```python
from build123d import *

# Parameters (mm, degrees)
SKETCH2_W           = 70
SKETCH2_H           = 140
SKETCH2_R           = 1.5
BOSS_EXTRUDE1_DEPTH = 3.175
SKETCH3_R           = 1.75
CUT_EXTRUDE1_DEPTH  = 79.326755486


with BuildPart() as part:
    # Sketch2 → Boss-Extrude1 (new body)
    with BuildSketch(Plane(origin=(0, 0, 0), x_dir=(1, 0, 0), z_dir=(0, 1, 0))):
        Rectangle(SKETCH2_W, SKETCH2_H)
        with Locations(Location((31, -62, 0), (0, 0, 270))):
            Circle(SKETCH2_R, mode=Mode.SUBTRACT)
        with Locations(Location((31, 62, 0), (0, 0, 90))):
            Circle(SKETCH2_R, mode=Mode.SUBTRACT)
        with Locations(Location((-31, 62, 0), (0, 0, 270))):
            Circle(SKETCH2_R, mode=Mode.SUBTRACT)
        with Locations(Location((-31, -62, 0), (0, 0, 90))):
            Circle(SKETCH2_R, mode=Mode.SUBTRACT)
    extrude(amount=BOSS_EXTRUDE1_DEPTH)

    # Sketch3 → Cut-Extrude1 (cut, through all)
    with BuildSketch(Plane(origin=(0, 3.175, 0), x_dir=(1, 0, 0), z_dir=(0, 1, 0))):
        with Locations(Location((-24.999549753, -44.6, 0), (0, 0, 270))):
            Circle(SKETCH3_R)
        with Locations(Location((24, -44.810057195, 0), (0, 0, 270))):
            Circle(SKETCH3_R)
        with Locations(Location((24, 13.189942805, 0), (0, 0, 90))):
            Circle(SKETCH3_R)
        with Locations(Location((-24.999549753, 12.97988561, 0), (0, 0, 90))):
            Circle(SKETCH3_R)
    extrude(amount=-CUT_EXTRUDE1_DEPTH, mode=Mode.SUBTRACT)


solid = part.part
```
Check sheet for the modelled part. Datum: model origin and axes. Units: mm. Round coordinates to 2 decimals unless told otherwise and drop trailing zeros. Loops run counter-clockwise (first coordinate to the right, second up) from the corner with the lowest first, then second, coordinate; pieces in that order, holes last. Notation, with made-up numbers: (78, 17.25) -> (120, 17.25) arc R20 ccw to (120, 43.25) -> close; hole circle Ø7 at (49, 22.25). An arc over 180 degrees is marked (long way). Answer in a Markdown table with one row per item.
Q1. Release check for a two-part mould opening along X. For faces 1 (the face through (0, 3.175, -1)), 2 (the face through (-35, 2, 1)), 3 (the face through (-25.67, 1.61, 46.217)), 4 (the face through (-23.29, 1.61, -12.6)) record: released by +X, released by -X, zero draft, split by the parting line, or undercut.
Data:
| item | result |
|---|---|
| face 1 | zero draft |
| face 2 | released by -X |
| face 3 | undercut |
| face 4 | undercut |
Q2. Sectioned sample at B-B on z = 62. Enter the section's corners in (x, y) (3 decimals).
Data:
| item | result |
|---|---|
| outline | (-35, 0) -> (-32.5, 0) -> (-32.5, 3.175) -> (-35, 3.175) -> close; (-29.5, 0) -> (29.5, 0) -> (29.5, 3.175) -> (-29.5, 3.175) -> close; (32.5, 0) -> (35, 0) -> (35, 3.175) -> (32.5, 3.175) -> close |
Q3. Thickness scan on L1, parallel to X at y = 1.4, z = 44.6; L2, parallel to X at y = 1.8, z = -62; L3, parallel to Z at x = -25, y = 0.85. Record the ranges inside material, lowest first.
Data:
| item | result |
|---|---|
| L1 | x = -35 to -26.75, -23.25 to 22.26, 25.74 to 35 |
| L2 | x = -35 to -32.5, -29.5 to 29.5, 32.5 to 35 |
| L3 | z = -70 to -14.73, -11.23 to 42.85, 46.35 to 70 |
Q4. Sectioned sample at A-A on x = 31. Enter the section's corners in (y, z) (3 decimals), then the cut area to 3 significant figures.
Data:
| item | result |
|---|---|
| outline | (0, -70) -> (3.175, -70) -> (3.175, -63.5) -> (0, -63.5) -> close; (0, -60.5) -> (3.175, -60.5) -> (3.175, 60.5) -> (0, 60.5) -> close; (0, 63.5) -> (3.175, 63.5) -> (3.175, 70) -> (0, 70) -> close |
| area | 425 mm^2 |
Q5. Go/stop test with a flat-tipped pin: P1, Ø2.5, axis at x = -31, z = 62, coming from the -Y side. Record where the tip stops, or that it passes through.
Data:
| item | result |
|---|---|
| P1 | passes through |
